For this review, use the dimensioned drawing (mm, ordinates from the lowest corner) and the shaded views. A direction names the side the tool comes from. Coordinates: 2 decimals unless noted, no trailing zeros. Loops run counter-clockwise (first coordinate to the right, second up) from the corner with the lowest first, then second, coordinate; pieces in that order, holes last. Notation, with made-up numbers: (10, 3.5) - (66, 3.5) arc R37 ccw to (66, 41.5) - close; hole circle Ø1 at (27, 55.25). An arc over 180 degrees is marked (long way). Answer in a Markdown table with one row per item. Add a question column.
(1) We need section A-A, the plane z = 10. Write out the cut boundary in (x, y).
(2) We need section D-D, the plane y = 3. Write out the cut boundary in (x, z), plus the area to 3 significant figures.
(3) We need section B-B, the plane x = 12. Write out the cut boundary in (y, z).
(4) To check wall thickness, follow L1, parallel to X at y = 9.25, z = 10.25; L2, parallel to Y at x = 19.45, z = 12.5; L3, parallel to X at y = 3.75, z = 16.25. State the ranges of each line that lie inside material, in increasing order. Write a range as [from, to].
(5) For the marked faces 1, 2 and 3, list the 3-axis set-ups (+Z, -Z, +X, -X, +Y, -Y) from which the entire face can be reached by the end or side of a thin tool; tool diameter is ignored.
(6) The part is to be moulded in two halves that separate along X. For the marked faces 4, 5, 6 and 7, say which applies: released by +X, released by -X, zero draft, split by the parting line, or undercut.
(7) Clearance check with flat-ended pins moving along their axes: pin 1 (8 mm diameter, centred on x = 10.5, z = 15, fed in from +Y); pin 2 (1.5 mm diameter, centred on y = 2, z = 17, fed in from -X); pin 3 (8 mm diameter, centred on x = 11, z = 4, fed in from -Y); pin 4 (4 mm diameter, centred on x = 4.5, z = 8, fed in from -Y). State where each tip first meets the part, or that it passes through.
(8) We need section C-C, the plane z = 12.5. Write out the cut boundary in (x, y), plus the area to 3 significant figures.
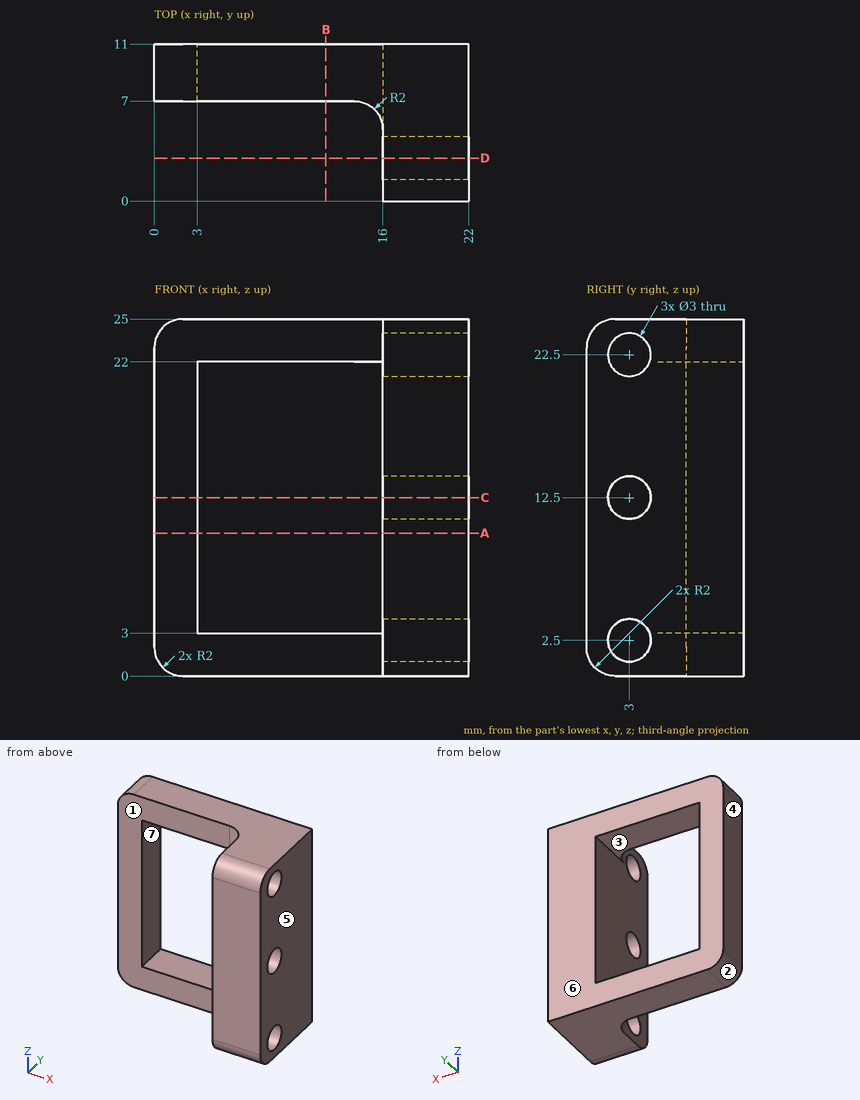
Responses:
| question | item | result |
|---|---|---|
| 1 | outline | (0, 7) - (3, 7) - (3, 11) - (0, 11) - close; (16, 0) - (22, 0) - (22, 11) - (16, 11) - close |
| 2 | outline | (16, 0) - (22, 0) - (22, 1) - (16, 1) - close; (16, 4) - (22, 4) - (22, 11) - (16, 11) - close; (16, 14) - (22, 14) - (22, 21) - (16, 21) - close; (16, 24) - (22, 24) - (22, 25) - (16, 25) - close |
| 2 | area | 96.0 mm2 |
| 3 | outline | (7, 0) - (11, 0) - (11, 3) - (7, 3) - close; (7, 22) - (11, 22) - (11, 25) - (7, 25) - close |
| 4 | L1 | x = [0, 3], [16, 22] |
| 4 | L2 | y = [0, 1.5], [4.5, 11] |
| 4 | L3 | x = [16, 22] |
| 5 | face 1 | +Z, -Z, -X, -Y |
| 5 | face 2 | -Z, -X, +Y, -Y |
| 5 | face 3 | +Y, -Y |
| 6 | face 4 | released by -X |
| 6 | face 5 | released by +X |
| 6 | face 6 | zero draft |
| 6 | face 7 | undercut |
| 7 | pin 1 | passes through |
| 7 | pin 2 | stops at x = 16 |
| 7 | pin 3 | stops at y = 6.8 |
| 7 | pin 4 | stops at y = 7 |
| 8 | outline | (0, 7) - (3, 7) - (3, 11) - (0, 11) - close; (16, 0) - (22, 0) - (22, 1.5) - (16, 1.5) - close; (16, 4.5) - (22, 4.5) - (22, 11) - (16, 11) - close |
| 8 | area | 60.0 mm2 |
